from build123d import *

# Parameters (mm, degrees)
SKETCH_1_R          = 4.1
EXTRUDE_1_DEPTH     = 32
SKETCH_3_R          = 1.35
SKETCH_3_W          = 23
SKETCH_3_H          = 12
CUT_EXTRUDE_1_DEPTH = 5
SKETCH_5_R          = 6
EXTRUDE_2_DEPTH     = 2
SKETCH_6_R          = 6
EXTRUDE_3_DEPTH     = 100
SKETCH_7_R          = 17.5
EXTRUDE_4_DEPTH     = 5
SKETCH_9_R          = 1.6
CUT_EXTRUDE_3_DEPTH = 140


with BuildPart() as part:
    # 草图1 → 凸台-拉伸1 (new body)
    with BuildSketch(Plane.XY):
        with BuildLine():
            Line((-32.405771928, 8.673637409), (-5.405771928, 8.673637409))
            Line((-5.405771928, 8.673637409), (0.594228072, 8.673637409))
            ThreePointArc((0.594228072, 8.673637409), (3.594228072, -2.522515014), (-4.601924351, 5.673637409))
            Line((-4.601924351, 5.673637409), (-29.405771928, 5.673637409))
            Line((-29.405771928, 5.673637409), (-29.405771928, -6.326362591))
            Line((-29.405771928, -6.326362591), (-32.405771928, -6.326362591))
            Line((-32.405771928, -6.326362591), (-32.405771928, 5.673637409))
            Line((-32.405771928, 5.673637409), (-32.405771928, 8.673637409))
        make_face()
        with Locations((0.594228072, 2.673637409)):
            Circle(SKETCH_1_R, mode=Mode.SUBTRACT)
    extrude(amount=EXTRUDE_1_DEPTH)

    # 草图3 → 切除-拉伸1 (cut)
    with BuildSketch(Plane.ZY.offset(32.405771928)):
        with Locations((29.75, -0.326362591)):
            Circle(SKETCH_3_R)
        with Locations((2.25, -0.326362591)):
            Circle(SKETCH_3_R)
        with Locations((16, -0.326362591)):
            Rectangle(SKETCH_3_W, SKETCH_3_H)
    extrude(amount=-CUT_EXTRUDE_1_DEPTH, mode=Mode.SUBTRACT)

    # 草图5 → 凸台-拉伸2 (add)
    with BuildSketch(Plane.XY.offset(32)):
        with Locations((0.594228072, 2.673637409)):
            Circle(SKETCH_5_R)
    extrude(amount=EXTRUDE_2_DEPTH)

    # 草图6 → 凸台-拉伸3 (add)
    with BuildSketch(Plane(origin=(0, 0, 0), x_dir=(-1, 0, 0), z_dir=(0, 0, -1))):
        with Locations((-0.594228072, 2.673637409)):
            Circle(SKETCH_6_R)
    extrude(amount=EXTRUDE_3_DEPTH)

    # 草图7 → 凸台-拉伸4 (add)
    with BuildSketch(Plane(origin=(0, 0, -100), x_dir=(-1, 0, 0), z_dir=(0, 0, -1))):
        with Locations((-0.594228072, 2.673637409)):
            Circle(SKETCH_7_R)
    extrude(amount=EXTRUDE_4_DEPTH)

    # 草图9 → 切除-拉伸3 (cut, through all)
    with BuildSketch(Plane(origin=(0, 0, -105), x_dir=(-1, 0, 0), z_dir=(0, 0, -1))):
        with Locations((11.905771928, 2.673637409)):
            Circle(SKETCH_9_R)
        with Locations((-0.594228072, 15.173637409)):
            Circle(SKETCH_9_R)
        with Locations((-13.094228072, 2.673637409)):
            Circle(SKETCH_9_R)
        with Locations((-0.594228072, -9.826362591)):
            Circle(SKETCH_9_R)
    extrude(amount=-CUT_EXTRUDE_3_DEPTH, mode=Mode.SUBTRACT)


solid = part.part
CAD build for the part. Positions are in the model's coordinates, mm. A direction names the side the tool comes from. Give positions to 0.01 mm unless a question says otherwise; leave off trailing zeros. Loops run counter-clockwise (first coordinate to the right, second up) from the corner with the lowest first, then second, coordinate; pieces in that order, holes last. Notation, with made-up numbers: M 13.5,72 L 69.5,72 A30 cw 69.5,107 Z; hole C 51.25,14.25 d1. An arc over 180 degrees is marked long. Answer in a Markdown table with one row per item. Add a question column.
Item 1: Tool access for faces 1 (the face through (-0.29, -1.33, 15.78)), 2 (the face through (-16, 8.674, 16)), 3 (the face through (-29.406, 1, 29)): list every direction of +Z, -Z, +X, -X, +Y, -Y with a clear straight run to the whole face (end or side of a thin tool).
Item 2: Probe probe 1 along Z at (x, y) = (1.5, -1); probe 2 along Y at (x, z) = (-30.25, 2.25); probe 3 along Z at (x, y) = (-15, -0.5). List the from-to ranges inside material, lowest first.
Item 3: Drop flat-ended pins along their axis: P1, Ø12, axis at x = -14.5, y = 3.5, coming from the +Z side; P2, Ø6, axis at x = -10, z = -24, coming from the +Y side; P3, Ø2, axis at y = -0.33, z = 2.25, coming from the -X side; P4, Ø1.5, axis at x = -31.5, y = -2.5, coming from the -Z side. Give the stop position or say it passes through.
Item 4: Mould opens along X. For faces 4 (the face through (-30.927, -1.644, 1.957)), 5 (the face through (-19, 5.674, 16)), 6 (the face through (1, 3, 0)), 7 (the face through (-15.57, -4.03, -102.46)) say: +X half, -X half, draft (parallel to the pull), parting line (faces both ways), or undercut.
Item 5: Band-saw the part on A-A on z = 2.25. Give the cut face in (x, y).
Reply:
| question | item | result |
|---|---|---|
| 1 | face 1 | none |
| 1 | face 2 | +Z, +X, -X, +Y |
| 1 | face 3 | +Z, -Z, -Y |
| 2 | probe 1 | z = -105 to 0, 32 to 34 |
| 2 | probe 2 | y = -6.33 to -1.68, 1.02 to 8.67 |
| 2 | probe 3 | z = -105 to -100 |
| 3 | P1 | stops at z = 32 |
| 3 | P2 | passes through |
| 3 | P3 | stops at x = -5.06 |
| 3 | P4 | stops at z = 0 |
| 4 | face 4 | draft |
| 4 | face 5 | undercut |
| 4 | face 6 | undercut |
| 4 | face 7 | parting line |
| 5 | outline | M -32.41,-6.33 L -29.41,-6.33 L -29.41,-1.68 L -32.41,-1.68 Z; M -32.41,1.02 L -29.41,1.02 L -29.41,5.67 L -4.6,5.67 A6 ccw long 0.59,8.67 L -32.41,8.67 Z; hole C 0.59,2.67 d8.2 |
